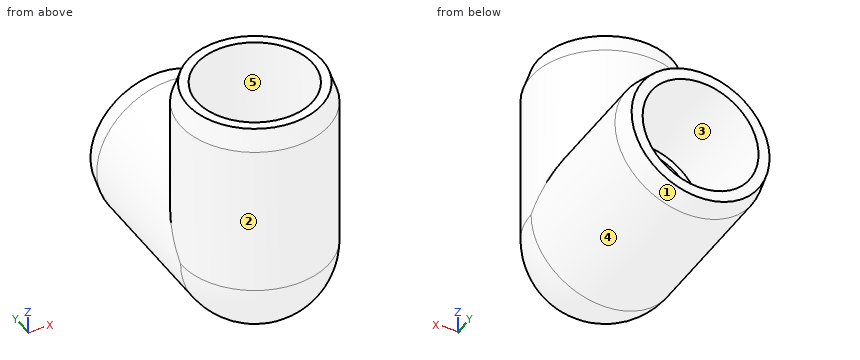
```python
from build123d import *

# Parameters (mm, degrees)
BOSS_EXTRUDE2_REACH      = 67.644
BOSS_EXTRUDE2_END_RADIUS = 13.6525
SKETCH5_R                = 13.6525
SKETCH5_R_2              = 10.668
SKETCH6_R                = 10.668
CUT_EXTRUDE1_DEPTH       = 43.688
CUT_EXTRUDE2_START       = 44.196
SKETCH7_R                = 10.668
CUT_EXTRUDE2_DEPTH       = 44.196
SKETCH8_W                = 1.27
SKETCH8_H                = 1.905
SKETCH9_W                = 1.905
SKETCH9_H                = 1.27


with BuildPart() as part:
    # Sketch2 → Revolve1 (revolve)
    with BuildSketch(Plane.XY):
        with BuildLine():
            Line((13.6525, 13.6525), (13.6525, 45.4025))
            Line((13.6525, 45.4025), (10.668, 45.4025))
            Line((10.668, 45.4025), (10.668, 13.6525))
            ThreePointArc((10.668, 13.6525), (7.543415142, 6.109084858), (0, 2.9845))
            Line((0, 2.9845), (0, 0))
            ThreePointArc((0, 0), (9.65377533, 3.99872467), (13.6525, 13.6525))
        make_face()
    revolve(axis=Axis((0, 50.454853333, 0), (0, -1, 0)))

    # Boss-Extrude2: up to this sphere (the profile starts outside it)
    boss_extrude2_end = Location((0, 13.6525, 0)) * Sphere(BOSS_EXTRUDE2_END_RADIUS, mode=Mode.PRIVATE)
    # Sketch5 → Boss-Extrude2 (add, up to the surface)
    with BuildSketch(Plane(origin=(0, 0, 31.75), x_dir=(-1, 0, 0), z_dir=(0, 0, -1)), mode=Mode.PRIVATE) as boss_extrude2_sk1:
        with Locations((0, 13.6525)):
            Circle(SKETCH5_R)
        with Locations((0, 13.6525)):
            Circle(SKETCH5_R_2, mode=Mode.SUBTRACT)
    boss_extrude2_tool1 = extrude(boss_extrude2_sk1.sketch, amount=BOSS_EXTRUDE2_REACH, mode=Mode.PRIVATE) - boss_extrude2_end
    add(boss_extrude2_tool1.solids().sort_by_distance((13.266349, 13.6525, 31.75))[0])

    # Sketch6 → Cut-Extrude1 (cut)
    with BuildSketch(Plane(origin=(0, 13.6525, 0), x_dir=(1, 0, 0), z_dir=(0, 1, 0))):
        with Locations(Location((0, 0, 0), (0, 0, 270))):
            Circle(SKETCH6_R)
    extrude(amount=CUT_EXTRUDE1_DEPTH, mode=Mode.SUBTRACT)

    # Sketch7 → Cut-Extrude2 (cut)
    with BuildSketch(Plane.XY.offset(CUT_EXTRUDE2_START)):
        with Locations(Location((0, 13.6525, 0), (0, 0, 180))):
            Circle(SKETCH7_R)
    extrude(amount=-CUT_EXTRUDE2_DEPTH, mode=Mode.SUBTRACT)

    # Sketch8 → Revolve2 (revolve)
    with BuildSketch(Plane.XY, mode=Mode.PRIVATE) as revolve2_sk:
        with Locations((-10.033, 25.4)):
            Rectangle(SKETCH8_W, SKETCH8_H)
    revolve(revolve2_sk.sketch.rotate(Axis((0, 45.4025, 0), (0, -1, 0)), 270), axis=Axis((0, 45.4025, 0), (0, -1, 0)))

    # Sketch9 → Revolve3 (revolve)
    with BuildSketch(Plane(origin=(0, 0, 0), x_dir=(0, 0, -1), z_dir=(1, 0, 0)), mode=Mode.PRIVATE) as revolve3_sk:
        with Locations((-11.7475, 3.6195)):
            Rectangle(SKETCH9_W, SKETCH9_H)
    revolve(revolve3_sk.sketch.rotate(Axis((0, 13.6525, 31.75), (0, 0, -1)), 270), axis=Axis((0, 13.6525, 31.75), (0, 0, -1)))

    # Sketch10 → Cut-Revolve1 (revolve, cut)
    with BuildSketch(Plane(origin=(0, 0, 0), x_dir=(0, 0, -1), z_dir=(1, 0, 0)), mode=Mode.PRIVATE) as cut_revolve1_sk:
        Polygon((13.6525, 45.4025), (13.6525, 41.5925), (12.7, 45.4025), align=None)
    revolve(cut_revolve1_sk.sketch.rotate(Axis((0, 45.4025, 0), (0, -1, 0)), 180), axis=Axis((0, 45.4025, 0), (0, -1, 0)), mode=Mode.SUBTRACT)

    # Sketch12 → Cut-Revolve2 (revolve, cut)
    with BuildSketch(Plane(origin=(0, 13.6525, 0), x_dir=(1, 0, 0), z_dir=(0, 1, 0)), mode=Mode.PRIVATE) as cut_revolve2_sk:
        Polygon((-13.6525, -31.75), (-13.6525, -27.94), (-12.3825, -31.75), align=None)
    revolve(cut_revolve2_sk.sketch.rotate(Axis((0, 13.6525, 31.75), (0, 0, -1)), 180), axis=Axis((0, 13.6525, 31.75), (0, 0, -1)), mode=Mode.SUBTRACT)


solid = part.part
```
For this review, take the finished solid that the model builds, in its own axes (mm). Face numbers are marked on the shaded views. A direction names the side the tool comes from. Round coordinates to 2 decimals unless told otherwise and drop trailing zeros. Write each loop counter-clockwise with the first axis right and the second up, starting at its lowest first coordinate (ties: lowest second). Pieces come first, ordered by that corner, then holes. Notation, with made-up numbers: (25.5, -17.75) - (77.5, -17.75) arc R17 cw to (77.5, 6.25) - close; hole circle Ø2 at (2.25, 27). An arc over 180 degrees is marked (long way). Use CSV: the item, a comma, the result in double quotes.
1) Wall thickness on line 1 along Z through (x, y) = (0, 39); line 2 along Y through (x, z) = (0, 11.7); line 3 along Y through (x, z) = (0.5, 10): over which ranges is each line inside the solid? List them lowest first. Write a range as from..to.
Conclusion:
line 1,"z = -13.65..-10.67, 10.67..13.65"
line 2,"y = 0..4.25, 23.05..45.4"
line 3,"y = 0.01..3, 24.45..26.35"
2) Add section B-B on y = 35. Write out the cut boundary in (x, z) (1 decimal), and give its area (3 significant figures).
Conclusion:
outline,"circle Ø27.3 at (0, 0); hole circle Ø21.3 at (0, 0)"
area,"228 mm^2"
3) For the marked faces 1 and 2, list the 3-axis set-ups (+Z, -Z, +X, -X, +Y, -Y) from which the entire face can be reached by the end or side of a thin tool; tool diameter is ignored.
Conclusion:
face 1,"+Y"
face 2,"+Z"
4) Add section C-C on z = 21. Write out the cut boundary in (x, y) (1 decimal), and give its area (3 significant figures).
Conclusion:
outline,"circle Ø27.3 at (0, 13.7); hole circle Ø21.3 at (0, 13.7)"
area,"228 mm^2"
5) The part is to be moulded in two halves that separate along Z. For the marked faces 3, 4 and 5, say which applies: pulls with the +Z half, pulls with the -Z half, needs draft (parallel to the pull), parting line crosses it, or undercut.
Conclusion:
face 3,"undercut"
face 4,"parting line crosses it"
face 5,"needs draft"
6) Clearance check with flat-ended pins moving along their axes: pin 1 Ø1 at (x, z) = (5, -6) entering from +Y; pin 2 Ø4 at (x, z) = (-6, 16) entering from +Y; pin 3 Ø12 at (y, z) = (40.5, 15.5) entering from -X. State where each tip first meets the part, or that it passes through.
Conclusion:
pin 1,"stops at y = 6.96"
pin 2,"stops at y = 26.71"
pin 3,"stops at x = -9.81"
